Geometry check sheet. Reference: the model listing, model coordinates, mm. A direction names the side the tool comes from. Coordinates: 2 decimals unless noted, no trailing zeros. Order: outer loops, then holes, each group sorted by start corner. A loop starts at its lowest first (then second) coordinate and runs counter-clockwise, first axis right, second up. Notation, with made-up numbers: (-7.75, 11.5) - (36.25, 11.5) arc R27 ccw to (36.25, 30.5) - close; hole circle Ø3 at (-26.5, 56.25). An arc over 180 degrees is marked (long way). Return JSON: item names as keys, results as strings. Group by question number.
Item 1: Section check A-A on z = 3.25. Enter the section's corners in (x, y), then the cut area to 3 significant figures.
Item 2: Draft check along X on faces 1 (the flat face through (15.14, -42.12, 3.55)), 2 (the flat face through (20, 0, 3)), 3 (the flat face through (-14.86, -42.88, 3.55)). Enter one of: pulls with the +X half, pulls with the -X half, needs draft (parallel to the pull), parting line crosses it, or undercut.
Item 3: Section check D-D on x = -21. Enter the section's corners in (y, z).
Item 4: Tool access check on faces 4 (the flat face through (0, -10, 3)), 5 (the flat face through (-22, 10, 3)). Record the directions out of +Z, -Z, +X, -X, +Y, -Y that give a thin tool (end or side, any length) a straight path to the whole face; none if there is none.
Item 5: Section check B-B on y = 3. Enter the section's corners in (x, z), then the cut area to 3 significant figures.
Item 6: Gauge pin test, flat ends, axial feed: pin 1 (3 mm diameter, centred on y = -52.5, z = 2.5, fed in from +X); pin 2 (2 mm diameter, centred on x = 4.5, z = 3, fed in from +Y). Record the tip position at first contact, or that the pin passes through.
Item 7: Section check C-C on x = 0. Enter the section's corners in (y, z).
Item 8: Scan lines: probe 1 along Y at (x, z) = (0, 5); probe 2 along X at (y, z) = (-65, 3.25); probe 3 along X at (y, z) = (-3, 3.5). Record each from-to range of solid material in increasing order.
from build123d import *

# Parameters (mm, degrees)
SALIENTE_EXTRUIR1_DEPTH = 7
CROQUIS2_W              = 10
CROQUIS2_H              = 10
CROQUIS2_R              = 1.1
SALIENTE_EXTRUIR2_DEPTH = 7


with BuildPart() as part:
    # Croquis1 → Saliente-Extruir1 (new body)
    with BuildSketch(Plane.XY):
        Polygon((-20, -10), (-20, 10), (-25, 10), (-25, -15), (25, -15), (25, 10), (20, 10), (20, -10), align=None)
    extrude(amount=SALIENTE_EXTRUIR1_DEPTH)

    # Croquis2 → Saliente-Extruir2 (add)
    # profile 1 of 2: a face of its own
    with BuildSketch(Plane.XY.offset(7)):
        Polygon((-5, -70), (-25, -15), (25, -15), (5, -70), (5, -60), (-5, -60), align=None)
    # profile 2 of 2: a face of its own
    with BuildSketch(Plane.XY.offset(7)):
        with Locations((0, -65)):
            Rectangle(CROQUIS2_W, CROQUIS2_H)
        with Locations((0, -65)):
            Circle(CROQUIS2_R, mode=Mode.SUBTRACT)
    extrude(amount=-SALIENTE_EXTRUIR2_DEPTH)


solid = part.part
Computed:
{
 "1": {"outline": "(-25, -15) - (-5, -70) - (5, -70) - (25, -15) - (25, 10) - (20, 10) - (20, -10) - (-20, -10) - (-20, 10) - (-25, 10) - close; hole circle Ø2.2 at (0, -65)", "area": "2,100 mm²"},
 "2": {"face 1": "pulls with the +X half", "face 2": "undercut", "face 3": "pulls with the -X half"},
 "3": {"outline": "(-26, 0) - (10, 0) - (10, 7) - (-26, 7) - close"},
 "4": {"face 4": "+Z, -Z, +Y", "face 5": "+Z, -Z, +X, -X, +Y"},
 "5": {"outline": "(-25, 0) - (-20, 0) - (-20, 7) - (-25, 7) - close; (20, 0) - (25, 0) - (25, 7) - (20, 7) - close", "area": "70.0 mm²"},
 "6": {"pin 1": "stops at x = 11.91", "pin 2": "stops at y = -10"},
 "7": {"outline": "(-70, 0) - (-66.1, 0) - (-66.1, 7) - (-70, 7) - close; (-63.9, 0) - (-10, 0) - (-10, 7) - (-63.9, 7) - close"},
 "8": {"probe 1": "y = -70 to -66.1, -63.9 to -10", "probe 2": "x = -6.82 to -1.1, 1.1 to 6.82", "probe 3": "x = -25 to -20, 20 to 25"}
}
